Here's how the part is built. I have some questions about the finished solid (model axes, mm). A direction names the side the tool comes from. Coordinates: 2 decimals unless noted, no trailing zeros.
Item 1: Please list where these lines run through material, in increasing order: line 1 (Z direction, x = 19, y = -52); line 2 (Z direction, x = 35, y = -120); line 3 (X direction, y = 3.5, z = -7.5).
Item 2: If we mould it in two halves opening along Z, with no side actions, what happens to faces 1 (the face through (0, -37, -5)), 2 (the face through (1.479, -9.824, -3.178))? For each: pulls with the +Z half, pulls with the -Z half, needs draft (parallel to the pull), parting line crosses it, or undercut.
Item 3: For faces 3 (the face through (1.479, -96.99, 2.464)), 4 (the face through (22, -105, 32)), which set-ups out of +Z, -Z, +X, -X, +Y, -Y let a thin tool reach every point of the face, with its end or its side?
Item 4: I'm going to push flat-ended pins straight in: P1, Ø0.9, axis at x = 1, y = -120, coming from the +Z side; P2, Ø13, axis at x = 20, y = 26, coming from the +Z side; P3, Ø3.5, axis at x = 15.5, z = 31, coming from the -Y side. Where does each tip first touch, or does it pass through?
from build123d import *

# Parameters (mm, degrees)
BOSS_EXTRUDE3_DEPTH  = 5
EXTRUDE_THIN3_DEPTH  = 35
RIB3_START           = -2.5
RIB3_DEPTH           = 5
RIB13_START          = -2.5
RIB13_DEPTH          = 5
LPATTERN1_COUNT      = 5
LPATTERN1_PITCH      = 30
MIRROR1_START        = -2.5
MIRROR1_COPY_1_DEPTH = 5
MIRROR1_COPY_2_DEPTH = 5
MIRROR1_COPY_3_DEPTH = 5
MIRROR1_COPY_4_DEPTH = 5
CUT_EXTRUDE1_START   = -40
SKETCH11_R           = 1
CUT_EXTRUDE1_DEPTH   = 10
FILLET2_R            = 10
SKETCH12_W           = 22
SKETCH12_H           = 1.974358974
CUT_EXTRUDE2_DEPTH   = 3


# Read off the part's stored shape, not the designer's step: Rib3, Rib13
with BuildPart() as part:
    # Sketch7 → Boss-Extrude3 (new body)
    with BuildSketch(Plane(origin=(0, 0, 0), x_dir=(0, 0, -1), z_dir=(1, 0, 0))):
        with BuildLine():
            Line((-34, 0), (-34, -150))
            ThreePointArc((-34, -150), (0, -143.330666624), (34, -150))
            Line((34, -150), (34, 0))
            ThreePointArc((34, 0), (0, 34), (-34, 0))
        make_face()
    extrude(amount=BOSS_EXTRUDE3_DEPTH)

    # Sketch10 → Extrude-Thin3 (add)
    with BuildSketch(Plane(origin=(5, 0, 0), x_dir=(0, 0, -1), z_dir=(1, 0, 0))):
        with BuildLine():
            Line((34, -150), (34, 0))
            ThreePointArc((34, 0), (0, 34), (-34, 0))
            Line((-34, 0), (-34, -150))
            ThreePointArc((-34, -150), (0, -143.330666624), (34, -150))
        make_face()
        with BuildLine():
            Line((32, -147.075232013), (32, 0))
            ThreePointArc((32, 0), (0, 32), (-32, 0))
            Line((-32, 0), (-32, -147.075232013))
            ThreePointArc((-32, -147.075232013), (0, -141.330666624), (32, -147.075232013))
        make_face(mode=Mode.SUBTRACT)
    extrude(amount=EXTRUDE_THIN3_DEPTH)

    # Rib3 outline → Rib3 (add)
    with BuildSketch(Plane.XY.offset(RIB3_START)):
        Polygon((5, 20), (40, 29), (40, 33), (4, 33), (4, 19.742857143), align=None)
    extrude(amount=RIB3_DEPTH)

    # Rib13 outline → Rib13 (add)
    with BuildSketch(Plane(origin=(0, 0, 0), x_dir=(1, 0, 0), z_dir=(0, 1, 0)).offset(RIB13_START)):
        Polygon((5, -32), (40, -32), (40, -30), (5, -29), align=None)
    rib13 = extrude(amount=RIB13_DEPTH)

    # LPattern1: Rib13 ×5
    with Locations(*[(0, -i * LPATTERN1_PITCH, 0) for i in range(1, LPATTERN1_COUNT)]):
        add(rib13)

    # Mirror1: Rib13 across plane
    add(rib13.mirror(Plane.XY))

    # Mirror1 copy 1 sketch → Mirror1 copy 1 (add)
    with BuildSketch(Plane(origin=(0, -30, 0), x_dir=(1, 0, 0), z_dir=(0, 1, 0)).offset(MIRROR1_START)):
        Polygon((5, 32), (40, 32), (40, 30), (5, 29), align=None)
    extrude(amount=MIRROR1_COPY_1_DEPTH)

    # Mirror1 copy 2 sketch → Mirror1 copy 2 (add)
    with BuildSketch(Plane(origin=(0, -60, 0), x_dir=(1, 0, 0), z_dir=(0, 1, 0)).offset(MIRROR1_START)):
        Polygon((5, 32), (40, 32), (40, 30), (5, 29), align=None)
    extrude(amount=MIRROR1_COPY_2_DEPTH)

    # Mirror1 copy 3 sketch → Mirror1 copy 3 (add)
    with BuildSketch(Plane(origin=(0, -90, 0), x_dir=(1, 0, 0), z_dir=(0, 1, 0)).offset(MIRROR1_START)):
        Polygon((5, 32), (40, 32), (40, 30), (5, 29), align=None)
    extrude(amount=MIRROR1_COPY_3_DEPTH)

    # Mirror1 copy 4 sketch → Mirror1 copy 4 (add)
    with BuildSketch(Plane(origin=(0, -120, 0), x_dir=(1, 0, 0), z_dir=(0, 1, 0)).offset(MIRROR1_START)):
        Polygon((5, 32), (40, 32), (40, 30), (5, 29), align=None)
    extrude(amount=MIRROR1_COPY_4_DEPTH)

    # Sketch11 → Cut-Extrude1 (cut)
    with BuildSketch(Plane.ZY.offset(CUT_EXTRUDE1_START)):
        with Locations(Location((-31.5, 0, 0), (0, 0, 180))):
            Circle(SKETCH11_R)
        with Locations(Location((31.5, 0, 0), (0, 0, 180))):
            Circle(SKETCH11_R)
        with Locations(Location((-31.5, -30, 0), (0, 0, 180))):
            Circle(SKETCH11_R)
        with Locations(Location((31.5, -30, 0), (0, 0, 180))):
            Circle(SKETCH11_R)
        with Locations(Location((-31.5, -60, 0), (0, 0, 180))):
            Circle(SKETCH11_R)
        with Locations(Location((31.5, -60, 0), (0, 0, 180))):
            Circle(SKETCH11_R)
        with Locations(Location((-31.5, -90, 0), (0, 0, 180))):
            Circle(SKETCH11_R)
        with Locations(Location((31.5, -90, 0), (0, 0, 180))):
            Circle(SKETCH11_R)
        with Locations(Location((-31.5, -120, 0), (0, 0, 180))):
            Circle(SKETCH11_R)
        with Locations(Location((31.5, -120, 0), (0, 0, 180))):
            Circle(SKETCH11_R)
        with Locations(Location((0, 31.5, 0), (0, 0, 180))):
            Circle(SKETCH11_R)
    extrude(amount=CUT_EXTRUDE1_DEPTH, mode=Mode.SUBTRACT)

    # Fillet2
    fillet2_edges = [part.edges().sort_by_distance(p)[0] for p in [
        (0, -75, -34),
        (0, -143.330666624, 0),
        (0, -75, 34),
        (0, 34, 0),
    ]]
    fillet(fillet2_edges, radius=FILLET2_R)

    # Sketch12 → Cut-Extrude2 (cut)
    # profile 1 of 7: a face of its own
    with BuildSketch(Plane.ZY):
        Polygon((-11, -1.692307692), (11, -4.596554487), (11, -4.878605769), (-7.051282051, -13.961538462), (11, -23.018028846), (11, -23.300080128), (-11, -26.230769231), (-11, -24.256410256), (4.816907051, -22.141025641), (-11, -14.203926282), (-11, -13.754407051), (4.865384615, -5.782051282), (-11, -3.679887821), align=None)
    # profile 2 of 7: a face of its own
    with BuildSketch(Plane.ZY):
        Polygon((11, -39.769230769), (-11, -49.923076923), (-11, -47.776842949), (-3.948717949, -44.524439103), (-3.948717949, -34.551282051), (-11, -31.210737179), (-11, -29.051282051), (11, -39.487179487), align=None)
        Polygon((6.707532051, -39.606169872), (-1.692307692, -35.626602564), (-1.692307692, -43.484375), align=None, mode=Mode.SUBTRACT)
    # profile 3 of 7: a face of its own
    with BuildSketch(Plane.ZY):
        with Locations((0, -54.294871795)):
            Rectangle(SKETCH12_W, SKETCH12_H)
    # profile 4 of 7: a face of its own
    with BuildSketch(Plane.ZY):
        Polygon((11, -68.538461538), (11, -70.512820513), (-8.743589744, -70.512820513), (-8.743589744, -78.974358974), (-11, -78.974358974), (-11, -68.538461538), align=None)
    # profile 5 of 7: a face of its own
    with BuildSketch(Plane.ZY):
        with Locations((0, -83.628205128)):
            Rectangle(SKETCH12_W, SKETCH12_H)
    # profile 6 of 7: a face of its own
    with BuildSketch(Plane.ZY):
        Polygon((-11, -89.41025641), (11, -89.41025641), (11, -89.824519231), (-6.315304487, -104.358974359), (11, -104.358974359), (11, -106.333333333), (-11, -106.333333333), (-11, -105.883814103), (6.275641026, -91.384615385), (-11, -91.384615385), align=None)
    # profile 7 of 7: a face of its own
    with BuildSketch(Plane.ZY):
        Polygon((11, -111.974358974), (11, -113.948717949), (1.974358974, -113.948717949), (1.974358974, -125.230769231), (11, -125.230769231), (11, -127.205128205), (-11, -127.205128205), (-11, -125.230769231), (-0.282051282, -125.230769231), (-0.282051282, -113.948717949), (-11, -113.948717949), (-11, -111.974358974), align=None)
    extrude(amount=-CUT_EXTRUDE2_DEPTH, mode=Mode.SUBTRACT)


solid = part.part
Answer:
1. line 1: z = -34 to -32, 32 to 34
1. line 2: z = -34 to -32.5, -30.5 to -29.86, 29.86 to 30.5, 32.5 to 34
1. line 3: x = 0 to 5
2. face 1: needs draft
2. face 2: undercut
3. face 3: -X
3. face 4: +X
4. P1: stops at z = 29.19
4. P2: stops at z = 27.85
4. P3: stops at y = -149.5
